Verification items for this drawing (mm, ordinates from the low corner). A direction names the side the tool comes from. Round coordinates to 2 decimals unless told otherwise and drop trailing zeros. Order: outer loops, then holes, each group sorted by start corner. A loop starts at its lowest first (then second) coordinate and runs counter-clockwise, first axis right, second up. Notation, with made-up numbers: (-15.75, -38.5) -> (28.25, -38.5) arc R18 ccw to (28.25, -30.5) -> close; hole circle Ø8 at (-37.5, -20). An arc over 180 degrees is marked (long way). Answer in a Markdown table with one row per item.
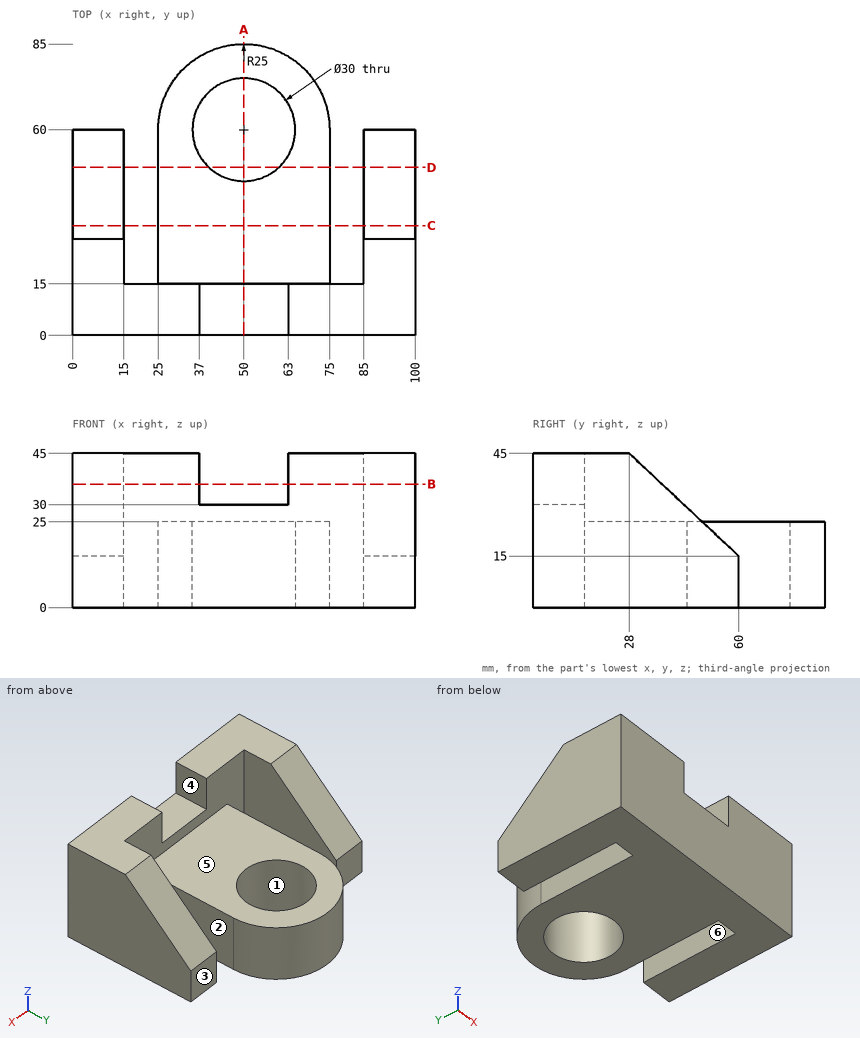
Item 1: Cross-section at A-A (x = 50). Record the boundary of the cut face in (y, z), and give its area (3 significant figures).
Result sheet:
| item | result |
|---|---|
| outline | (0, 0) -> (45, 0) -> (45, 25) -> (15, 25) -> (15, 30) -> (0, 30) -> close; (75, 0) -> (85, 0) -> (85, 25) -> (75, 25) -> close |
| area | 1,450 mm^2 |
Item 2: Scan lines: line 1 (X direction, y = 38, z = 13); line 2 (Y direction, x = 50, z = 17); line 3 (Y direction, x = 39.5, z = 21). Record each from-to range of solid material in increasing order. Write a range as [from, to].
Result sheet:
| item | result |
|---|---|
| line 1 | x = [0, 15], [25, 75], [85, 100] |
| line 2 | y = [0, 45], [75, 85] |
| line 3 | y = [0, 49.29], [70.71, 82.69] |
Item 3: Set-up check for the marked faces 4, 5 and 6: record each of +Z, -Z, +X, -X, +Y, -Y from which the full face is reachable in a straight line by a thin tool's end or side.
Result sheet:
| item | result |
|---|---|
| face 4 | +Z, +Y, -Y |
| face 5 | +Z, +Y |
| face 6 | +Z, -Z, +Y |
Item 4: Depth check by flat-ended pin: P1, Ø8, axis at x = 23.5, z = 6.5, coming from the +Y side; P2, Ø25, axis at x = 49, y = 37.5, coming from the +Z side; P3, Ø12, axis at x = 7, z = 8.5, coming from the +Y side. Enter the tip coordinate at first touch or a pass-through.
Result sheet:
| item | result |
|---|---|
| P1 | stops at y = 70.9 |
| P2 | stops at z = 25 |
| P3 | stops at y = 60 |
Item 5: Mould release check, pull along Y, two halves, no side actions. Record for the marked faces 1, 2 and 3: pulls with the +Y half, pulls with the -Y half, needs draft (parallel to the pull), parting line crosses it, or undercut.
Result sheet:
| item | result |
|---|---|
| face 1 | undercut |
| face 2 | needs draft |
| face 3 | pulls with the +Y half |
Item 6: Cross-section at B-B (z = 36). Record the boundary of the cut face in (x, y).
Result sheet:
| item | result |
|---|---|
| outline | (0, 0) -> (37, 0) -> (37, 15) -> (15, 15) -> (15, 37.6) -> (0, 37.6) -> close; (63, 0) -> (100, 0) -> (100, 37.6) -> (85, 37.6) -> (85, 15) -> (63, 15) -> close |
Item 7: Cross-section at D-D (y = 49). Record the boundary of the cut face in (x, z), and give its area (3 significant figures).
Result sheet:
| item | result |
|---|---|
| outline | (0, 0) -> (15, 0) -> (15, 25.31) -> (0, 25.31) -> close; (25, 0) -> (39.8, 0) -> (39.8, 25) -> (25, 25) -> close; (60.2, 0) -> (75, 0) -> (75, 25) -> (60.2, 25) -> close; (85, 0) -> (100, 0) -> (100, 25.31) -> (85, 25.31) -> close |
| area | 1,500 mm^2 |
Item 8: Cross-section at C-C (y = 32). Record the boundary of the cut face in (x, z), and give its area (3 significant figures).
Result sheet:
| item | result |
|---|---|
| outline | (0, 0) -> (15, 0) -> (15, 41.25) -> (0, 41.25) -> close; (25, 0) -> (75, 0) -> (75, 25) -> (25, 25) -> close; (85, 0) -> (100, 0) -> (100, 41.25) -> (85, 41.25) -> close |
| area | 2,490 mm^2 |
